Autodesk Inventor part; units mm, degrees
ref_plane "YZ Plane" through (0, 0, 0) normal (1, 0, 0) x (0, 1, 0)
ref_plane "XZ Plane" through (0, 0, 0) normal (0, 1, 0) x (-1, 0, 0)
ref_plane "XY Plane" through (0, 0, 0) normal (0, 0, 1) x (1, 0, 0)
sketch "Sketch1" plane through (0, 0, 0) normal (0, 1, 0) x (-1, 0, 0)
  circle A0 centre (0, 0) radius 7.9
  circle A1 centre (0, 0) radius 5.85
  circle A2 centre (0, 0) radius 1.5
  dimension "d0" = 15.8
  dimension "d1" = 11.7
  dimension "d3" = 3
extrude "Extrusion1" add sketch "Sketch1" along normal blind 1.5 contours A0 | A1
extrude "Extrusion2" add sketch "Sketch1" along normal blind 6 contours A1
fillet "Fillet1" radius 0.75 1 edges at (5.85, 6, 0)
properties part number "juki-nozzle-base"
Could you check a few things on this model? Use its own coordinates, in mm. A direction names the side the tool comes from. Give positions to 0.01 mm unless a question says otherwise; leave off trailing zeros. Loops run counter-clockwise (first coordinate to the right, second up) from the corner with the lowest first, then second, coordinate; pieces in that order, holes last. Notation, with made-up numbers: (76, 62) -> (95, 62) arc R17 ccw to (95, 78) -> close; hole circle Ø2 at (30, 27). An arc over 180 degrees is marked (long way). Return JSON: item names as keys, results as strings.
Item 1: I'm going to push flat-ended pins straight in: pin 1 (4 mm diameter, centred on x = 0, z = 0, fed in from +Y); pin 2 (1 mm diameter, centred on x = -5, z = -6, fed in from +Y); pin 3 (3 mm diameter, centred on x = -0.5, y = 3.5, fed in from +Z); pin 4 (1.5 mm diameter, centred on y = 3.5, z = 2, fed in from -X). Where does each tip first touch, or does it pass through?
Geometry results:
{"pin 1": "stops at y = 6", "pin 2": "stops at y = 1.5", "pin 3": "stops at z = 5.85", "pin 4": "stops at x = -5.71"}
Item 2: If we section it at A-A on z = 0: List the corners of the cut face in (x, y) for me, plus the area to 3 significant figures.
Geometry results:
{"outline": "(-7.9, 0) -> (-1.5, 0) -> (-1.5, 6) -> (-5.1, 6) arc R0.75 ccw to (-5.85, 5.25) -> (-5.85, 1.5) -> (-7.9, 1.5) -> close; (1.5, 0) -> (7.9, 0) -> (7.9, 1.5) -> (5.85, 1.5) -> (5.85, 5.25) arc R0.75 ccw to (5.1, 6) -> (1.5, 6) -> close", "area": "58.1 mm²"}
Item 3: If we section it at B-B on x = 0: List the corners of the cut face in (y, z) for me, plus the area to 3 significant figures.
Geometry results:
{"outline": "(0, -7.9) -> (1.5, -7.9) -> (1.5, -5.85) -> (5.25, -5.85) arc R0.75 ccw to (6, -5.1) -> (6, -1.5) -> (0, -1.5) -> close; (0, 1.5) -> (6, 1.5) -> (6, 5.1) arc R0.75 ccw to (5.25, 5.85) -> (1.5, 5.85) -> (1.5, 7.9) -> (0, 7.9) -> close", "area": "58.1 mm²"}
Item 4: We'd pull the mould along X, two halves only. Please class faces 3 (the cylindrical face through (1.5, 2.96, -0.07)), 4 (the flat face through (1.2, 6, 1.2)), 5 (the cylindrical face through (6.269, 0.74, 4.807)): +X half, -X half, draft (parallel to the pull), parting line (faces both ways), or undercut.
Geometry results:
{"face 3": "undercut", "face 4": "draft", "face 5": "parting line"}
Item 5: Which directions (+Z, -Z, +X, -X, +Y, -Y) give clear straight access to the entire face, cutting with the end or side of a thin tool? Please do faces 1 (the flat face through (0, 0, -2)), 2 (the flat face through (6, 1.5, 0)).
Geometry results:
{"face 1": "+Z, -Z, +X, -X, -Y", "face 2": "+Y"}
Item 6: I need wall thicknesses on L1, parallel to Z at x = 0, y = 1.25; L2, parallel to Z at x = 0, y = 3.6; L3, parallel to Y at x = -3.25, z = -6. Which ranges of each line are inside material? Lowest first, please. Write a range as from..to.
Geometry results:
{"L1": "z = -7.9..-1.5, 1.5..7.9", "L2": "z = -5.85..-1.5, 1.5..5.85", "L3": "y = 0..1.5"}
Item 7: If we section it at D-D on y = 1.8: List the corners of the cut face in (x, z) for me.
Geometry results:
{"outline": "circle Ø11.7 at (0, 0); hole circle Ø3 at (0, 0)"}
Item 8: If we section it at C-C on y = 0.75: List the corners of the cut face in (x, z) for me.
Geometry results:
{"outline": "circle Ø15.8 at (0, 0); hole circle Ø3 at (0, 0)"}
